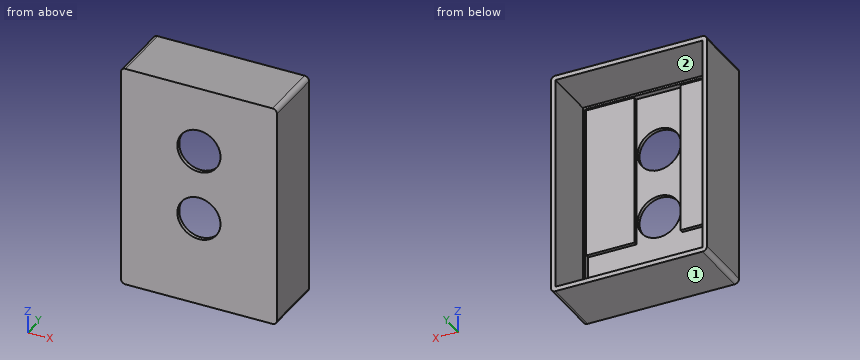
from build123d import *

# Parameters (mm, degrees)
SKETCH1_W           = 86.36
SKETCH1_H           = 124.333
BOSS_EXTRUDE1_DEPTH = 34.6202
SKETCH3_W           = 78.74
SKETCH3_H           = 116.84
CUT_EXTRUDE1_DEPTH  = 30.5816
SKETCH4_W           = 81.28
SKETCH4_H           = 119.253
CUT_EXTRUDE2_DEPTH  = 29.464
CUT_EXTRUDE3_DEPTH  = 2.032
SKETCH8_R           = 11.938
CUT_EXTRUDE4_DEPTH  = 2.032
FILLET1_R           = 2.54


with BuildPart() as part:
    # Sketch1 → Boss-Extrude1 (new body)
    with BuildSketch(Plane(origin=(0, 0, 0), x_dir=(1, 0, 0), z_dir=(0, 1, 0))):
        with Locations((43.18, 62.1665)):
            Rectangle(SKETCH1_W, SKETCH1_H)
    extrude(amount=BOSS_EXTRUDE1_DEPTH)

    # Sketch3 → Cut-Extrude1 (cut)
    with BuildSketch(Plane(origin=(0, 34.6202, 0), x_dir=(1, 0, 0), z_dir=(0, 1, 0))):
        with Locations((43.18, 62.23)):
            Rectangle(SKETCH3_W, SKETCH3_H)
    extrude(amount=-CUT_EXTRUDE1_DEPTH, mode=Mode.SUBTRACT)

    # Sketch4 → Cut-Extrude2 (cut)
    with BuildSketch(Plane(origin=(0, 34.6202, 0), x_dir=(1, 0, 0), z_dir=(0, 1, 0))):
        with Locations((43.18, 62.1665)):
            Rectangle(SKETCH4_W, SKETCH4_H)
    extrude(amount=-CUT_EXTRUDE2_DEPTH, mode=Mode.SUBTRACT)

    # Sketch6 → Cut-Extrude3 (cut)
    with BuildSketch(Plane(origin=(0, 4.0386, 0), x_dir=(1, 0, 0), z_dir=(0, 1, 0))):
        Polygon((3.81, 120.65), (82.55, 120.65), (82.55, 87.471955448), (55.88, 87.471955448), (55.88, 3.81), (30.48, 3.81), (30.48, 87.471955448), (3.81, 87.471955448), align=None)
    extrude(amount=-CUT_EXTRUDE3_DEPTH, mode=Mode.SUBTRACT)

    # Sketch8 → Cut-Extrude4 (cut)
    with BuildSketch(Plane(origin=(0, 2.0066, 0), x_dir=(1, 0, 0), z_dir=(0, 1, 0))):
        with Locations(Location((43.18, 36.1188, 0), (0, 0, 270))):
            Circle(SKETCH8_R)
        with Locations(Location((43.18, 74.93, 0), (0, 0, 270))):
            Circle(SKETCH8_R)
    extrude(amount=-CUT_EXTRUDE4_DEPTH, mode=Mode.SUBTRACT)

    # Fillet1
    fillet1_edges = [part.edges().sort_by_distance(p)[0] for p in [
        (86.36, 17.3101, 0),
        (0, 17.3101, 0),
        (0, 17.3101, -124.333),
        (86.36, 17.3101, -124.333),
    ]]
    fillet(fillet1_edges, radius=FILLET1_R)


solid = part.part
Could you check a few things on this model? Use its own coordinates, in mm. Face numbers are marked on the shaded views. A direction names the side the tool comes from. Give positions to 0.01 mm unless a question says otherwise; leave off trailing zeros. Loops run counter-clockwise (first coordinate to the right, second up) from the corner with the lowest first, then second, coordinate; pieces in that order, holes last. Notation, with made-up numbers: (59, 37) -> (81, 37) arc R26 ccw to (81, 57) -> close; hole circle Ø1 at (51.25, -38). An arc over 180 degrees is marked (long way). Return JSON: item names as keys, results as strings.
Item 1: If we section it at D-D on z = -100: List the corners of the cut face in (x, y) for me.
Geometry results:
{"outline": "(0, 0) -> (86.36, 0) -> (86.36, 34.62) -> (83.82, 34.62) -> (83.82, 5.16) -> (82.55, 5.16) -> (82.55, 2.01) -> (3.81, 2.01) -> (3.81, 5.16) -> (2.54, 5.16) -> (2.54, 34.62) -> (0, 34.62) -> close"}
Item 2: If we section it at A-A on x = 43.18: List the corners of the cut face in (y, z) for me, plus the area to 3 significant figures.
Geometry results:
{"outline": "(0, -124.33) -> (34.62, -124.33) -> (34.62, -121.79) -> (5.16, -121.79) -> (5.16, -120.65) -> (2.01, -120.65) -> (2.01, -86.87) -> (0, -86.87) -> close; (0, -62.99) -> (2.01, -62.99) -> (2.01, -48.06) -> (0, -48.06) -> close; (0, -24.18) -> (2.01, -24.18) -> (2.01, -3.81) -> (5.16, -3.81) -> (5.16, -2.54) -> (34.62, -2.54) -> (34.62, 0) -> (0, 0) -> close", "area": "327 mm²"}
Item 3: Which directions (+Z, -Z, +X, -X, +Y, -Y) give clear straight access to the entire face, cutting with the end or side of a thin tool? Please do the marked faces 1 and 2.
Geometry results:
{"face 1": "-Z, +X, -X, +Y, -Y", "face 2": "+Y"}
Item 4: I need wall thicknesses on L1, parallel to X at y = 15, z = -87; L2, parallel to X at y = 1.55, z = -74.93; L3, parallel to Z at x = 54.5, y = 8. Which ranges of each line are inside material? Lowest first, please. Write a range as from..to.
Geometry results:
{"L1": "x = 0..2.54, 83.82..86.36", "L2": "x = 0..31.24, 55.12..86.36", "L3": "z = -124.33..-121.79, -2.54..0"}
Item 5: I'm going to push a flat-ended pin straight in: pin 1 (3 mm diameter, centred on x = 71, z = -63.5, fed in from +Y). Where does the tip first touch, or does it pass through?
Geometry results:
{"pin 1": "stops at y = 4.04"}
Item 6: If we section it at B-B on z = -74.93: List the corners of the cut face in (x, y) for me, plus the area to 3 significant figures.
Geometry results:
{"outline": "(0, 0) -> (31.24, 0) -> (31.24, 2.01) -> (30.48, 2.01) -> (30.48, 4.04) -> (3.81, 4.04) -> (3.81, 5.16) -> (2.54, 5.16) -> (2.54, 34.62) -> (0, 34.62) -> close; (55.12, 0) -> (86.36, 0) -> (86.36, 34.62) -> (83.82, 34.62) -> (83.82, 5.16) -> (82.55, 5.16) -> (82.55, 4.04) -> (55.88, 4.04) -> (55.88, 2.01) -> (55.12, 2.01) -> close", "area": "407 mm²"}
Item 7: If we section it at C-C on y = 9: List the corners of the cut face in (x, z) for me, plus the area to 3 significant figures.
Geometry results:
{"outline": "(0, -121.79) arc R2.54 ccw to (2.54, -124.33) -> (83.82, -124.33) arc R2.54 ccw to (86.36, -121.79) -> (86.36, -2.54) arc R2.54 ccw to (83.82, 0) -> (2.54, 0) arc R2.54 ccw to (0, -2.54) -> close; hole (2.54, -121.79) -> (83.82, -121.79) -> (83.82, -2.54) -> (2.54, -2.54) -> close", "area": "1,040 mm²"}
